Design review of the part built by this model. Coordinates are the model's own, in mm. A direction names the side the tool comes from. Give positions to 0.01 mm unless a question says otherwise; leave off trailing zeros. Write each loop counter-clockwise with the first axis right and the second up, starting at its lowest first coordinate (ties: lowest second). Pieces come first, ordered by that corner, then holes.
Autodesk Inventor part; units mm, degrees
ref_plane "YZ Plane" through (0, 0, 0) normal (1, 0, 0) x (0, 1, 0)
ref_plane "XZ Plane" through (0, 0, 0) normal (0, 1, 0) x (-1, 0, 0)
ref_plane "XY Plane" through (0, 0, 0) normal (0, 0, 1) x (1, 0, 0)
sketch "スケッチ1" plane through (0, 0, 0) normal (1, 0, 0) x (0, 1, 0)
  line L0 (-5, -25) -> (5, -25)
  line L1 (5, -25) -> (5, 25)
  line L2 (5, 25) -> (-5, 25)
  line L3 (-5, 25) -> (-5, -25)
  line L4 (-5, -25) -> (5, 25) construction
  line L5 (5, -25) -> (-5, 25) construction
  line L6 (5, 25) -> (22.5, 25)
  line L7 (22.5, 25) -> (22.5, -25)
  line L8 (22.5, -25) -> (5, -25)
  line L9 (5, -25) -> (5, 25)
  point P0 (0, 0)
  dimension "d0" = 10
  dimension "d1" = 50
  dimension "d2" = 17.5
extrude "押し出し1" add sketch "スケッチ1" along normal blind 3
sketch "スケッチ2" plane through (3, 0, 0) normal (1, 0, 0) x (0, 0, -1)
  line L0 (25, -5) -> (25, 22.5)
  line L1 (25, 22.5) -> (-25, 22.5)
  point P0 (0, 0)
  point P1 (-20, 0)
  point P2 (20, 0)
  point P3 (-20, 18)
  point P4 (0, 18)
  point P5 (20, 18)
  dimension "d5" = 40
  dimension "d6" = 5
  dimension "d7" = 4.5
  dimension "d28" = 4.5
  dimension "d29" = 4.5
hole "穴1" at (3, 0, 20) at (3, 0, -20) at (3, 18, 20) at (3, 18, 0) at (3, 18, -20) direction (-1, 0, 0) diameter 3.2 end through all
sketch "スケッチ3" plane through (0, 0, 0) normal (-1, 0, 0) x (0, 0, 1)
  circle A0 centre (-20, 0) radius 1.6
  circle A1 centre (-20, 0) radius 3
  circle A2 centre (20, 0) radius 1.6
  circle A3 centre (20, 0) radius 3
  point P0 (0, 0)
  dimension "d15" = 6
  dimension "d16" = 6
extrude "押し出し2" cut sketch "スケッチ3" against normal blind 1 contours A0 | A1 | A2 | A3
sketch "スケッチ4" plane through (0, 0, 0) normal (-1, 0, 0) x (0, 0, 1)
  circle A0 centre (-20, 18) radius 1.6
  circle A1 centre (-20, 18) radius 3
  circle A2 centre (0, 18) radius 1.6
  circle A3 centre (0, 18) radius 3
  circle A4 centre (20, 18) radius 1.6
  circle A5 centre (20, 18) radius 3
  point P0 (0, 0)
  dimension "d19" = 6
  dimension "d20" = 6
  dimension "d21" = 6
extrude "押し出し3" cut sketch "スケッチ4" against normal blind 1 contours A0 | A1 | A3 | A4 | A5
sketch "スケッチ5" plane through (0, 0, 0) normal (-1, 0, 0) x (0, 0, 1)
  line L0 (15, 5) -> (-15, 5)
  line L1 (-15, 5) -> (-15, -5)
  line L2 (-15, -5) -> (15, -5)
  line L3 (15, -5) -> (15, 5)
  line L4 (15, 5) -> (-15, -5) construction
  line L5 (-15, 5) -> (15, -5) construction
  point P0 (0, 0)
  dimension "d24" = 30
  dimension "d25" = 10
extrude "押し出し4" cut sketch "スケッチ5" against normal blind 3
properties part number "stopper"
(1) Consider section B-B, the plane z = 0. Give the boundary of the cut face in (x, y).
Resolved:
outline: (0, 5) - (3, 5) - (3, 16.4) - (1, 16.4) - (1, 15) - (0, 15) - close; (0, 21) - (1, 21) - (1, 19.6) - (3, 19.6) - (3, 22.5) - (0, 22.5) - close
(2) Consider section C-C, the plane z = 20. Give the boundary of the cut face in (x, y), then the cut area to 3 significant figures.
Resolved:
outline: (0, -5) - (3, -5) - (3, -1.6) - (1, -1.6) - (1, -3) - (0, -3) - close; (0, 3) - (1, 3) - (1, 1.6) - (3, 1.6) - (3, 16.4) - (1, 16.4) - (1, 15) - (0, 15) - close; (0, 21) - (1, 21) - (1, 19.6) - (3, 19.6) - (3, 22.5) - (0, 22.5) - close
area: 57.7 mm2
(3) Mouldability with a two-part tool opening along Y and no side actions: class faces 1 (the face through (1, -5, -20)), 2 (the face through (1, 0, 15)), 3 (the face through (1.986, 16.414, 0.208)) as pulls with the +Y half, pulls with the -Y half, needs draft (parallel to the pull), parting line crosses it, or undercut.
Resolved:
face 1: pulls with the -Y half
face 2: needs draft
face 3: undercut
(4) To check wall thickness, follow L1, parallel to Z at x = 1.6, y = 18; L2, parallel to Y at x = 0.75, z = -20; L3, parallel to Z at x = 0.55, y = 18.25. State the ranges of each line that lie inside material, in increasing order.
Resolved:
L1: z = -25 to -21.6, -18.4 to -1.6, 1.6 to 18.4, 21.6 to 25
L2: y = -5 to -3, 3 to 15, 21 to 22.5
L3: z = -25 to -22.99, -17.01 to -2.99, 2.99 to 17.01, 22.99 to 25
(5) Consider section A-A, the plane x = 2.45. Give the boundary of the cut face in (y, z).
Resolved:
outline: (-5, -25) - (22.5, -25) - (22.5, 25) - (-5, 25) - (-5, 15) - (5, 15) - (5, -15) - (-5, -15) - close; hole circle Ø3.2 at (0, -20); hole circle Ø3.2 at (0, 20); hole circle Ø3.2 at (18, -20); hole circle Ø3.2 at (18, 0); hole circle Ø3.2 at (18, 20)
(6) Consider section D-D, the plane z = -13. Give the boundary of the cut face in (x, y).
Resolved:
outline: (0, 5) - (3, 5) - (3, 22.5) - (0, 22.5) - close
(7) Clearance check with flat-ended pins moving along their axes: P1, Ø2.5, axis at y = 18, z = 20, coming from the +X side; P2, Ø3.5, axis at y = 0, z = -20, coming from the -X side; P3, Ø1.5, axis at x = 2, z = -3.5, coming from the -Y side. State where each tip first meets the part, or that it passes through.
Resolved:
P1: passes through
P2: stops at x = 1
P3: stops at y = 5
(8) Tool access review of faces 4 (the face through (1, -1.3, 21.3)), 5 (the face through (1, 22.5, 0)): name each direction out of +Z, -Z, +X, -X, +Y, -Y from which nothing blocks a thin tool from reaching the whole face with its end or side.
Resolved:
face 4: -X
face 5: +Z, -Z, +X, -X, +Y
